For this review, take the finished solid that the model builds, in its own axes (mm). Round coordinates to 2 decimals unless told otherwise and drop trailing zeros. Order: outer loops, then holes, each group sorted by start corner. A loop starts at its lowest first (then second) coordinate and runs counter-clockwise, first axis right, second up. Notation, with made-up numbers: M 76.25,-8.75 L 108.25,-8.75 A11 ccw 108.25,4.25 Z; hole C 12.5,32 d6. An arc over 180 degrees is marked long. Answer as a JSON object with one key per item and string values.
from build123d import *

# Parameters (mm, degrees)
F0_R     = 1.98
F0_W     = 156.2984559469
F0_H     = 16.9940508366
F1_DEPTH = 2
F2_DEPTH = 3.81
F3_DEPTH = 44.45


with BuildPart() as f1:
    # F0 (on Top) → F1 (new body)
    with BuildSketch(Plane.XY):
        Polygon((-6.99, 165.1), (-6.99, -5.08), (163.2, -5.08), (163.2, 148.1059491634), (6.9015440531, 148.1059491634), (6.9015440531, 165.1), align=None)
        Circle(F0_R, mode=Mode.SUBTRACT)
        with Locations((157.48, 0)):
            Circle(F0_R, mode=Mode.SUBTRACT)
        with Locations((0, 154.94)):
            Circle(F0_R, mode=Mode.SUBTRACT)
        with Locations((157.48, 132.08)):
            Circle(F0_R, mode=Mode.SUBTRACT)
        with Locations((85.0507720266, 156.6029745817)):
            Rectangle(F0_W, F0_H)
    extrude(amount=-F1_DEPTH)

    # F0 (on Top) → F2 (join)
    with BuildSketch(Plane.XY):
        with Locations((85.0507720266, 156.6029745817)):
            Rectangle(F0_W, F0_H)
        Polygon((163.2, 165.1), (163.2, 148.1059491634), (165.6916588545, 148.1059491634), (165.6916588545, 167.9547131062), (6.9015440531, 167.9547131062), (6.9015440531, 165.1), align=None)
    extrude(amount=-F2_DEPTH)

    # F3 (add): a face of the model
    f3_faces = [f1.faces().sort_by_distance(p)[0] for p in [
        (86.2966014538, 158.0303311348, -3.81),
    ]]
    extrude(f3_faces, amount=-F3_DEPTH)


solid = f1.part
1) Add section B-B on y = 41.5. State the section outline as (x, z) points, and give its area (3 significant figures).
Geometry check:
{"outline": "M -6.99,-2 L 163.2,-2 L 163.2,0 L -6.99,0 Z", "area": "340 mm²"}
2) Add section C-C on z = 20. State the section outline as (x, y) points.
Geometry check:
{"outline": "M 6.9,148.11 L 165.69,148.11 L 165.69,167.95 L 6.9,167.95 Z"}
3) Insertion check: P1, Ø4, axis at x = 74.5, z = 33.5, coming from the -Y side; P2, Ø5, axis at x = 157.48, y = 0, coming from the +Z side; P3, Ø4.5, axis at x = 0, y = 0, coming from the -Z side. Each pin has a flat end and moves straight along its axis. Give the tip position at first contact, or say it passes through.
Geometry check:
{"P1": "stops at y = 148.11", "P2": "stops at z = 0", "P3": "stops at z = -2"}
4) Add section A-A on x = 153.5. State the section outline as (y, z) points.
Geometry check:
{"outline": "M -5.08,-2 L 148.11,-2 L 148.11,-3.81 L 167.95,-3.81 L 167.95,40.64 L 148.11,40.64 L 148.11,0 L -5.08,0 Z"}
5) For L1, parallel to Y at x = 157.48, z = -1.35; L2, parallel to Y at x = 0, z = -1; L3, parallel to X at y = 154.94, z = -0.6, list the stretches that pass through material, from the lowest coordinate up.
Geometry check:
{"L1": "y = -5.08 to -1.98, 1.98 to 130.1, 134.06 to 167.95", "L2": "y = -5.08 to -1.98, 1.98 to 152.96, 156.92 to 165.1", "L3": "x = -6.99 to -1.98, 1.98 to 165.69"}
6) Mouldability with a two-part tool opening along Y and no side actions: class faces 1 (the flat face through (85, 158, -3.81)), 2 (the flat face through (87, 167.955, 19)), 3 (the cylindrical face through (-0.429, -1.933, -0.986)) as +Y half, -Y half, draft (parallel to the pull), parting line (faces both ways), or undercut.
Geometry check:
{"face 1": "draft", "face 2": "+Y half", "face 3": "undercut"}
